Geometry: see drawing. Coordinates: mm, zero at the bounding-box minimum. Round coordinates to 2 decimals unless told otherwise and drop trailing zeros. Loops run counter-clockwise (first coordinate to the right, second up) from the corner with the lowest first, then second, coordinate; pieces in that order, holes last.
(1) Cut plane C-C, the plane z = 28.5. Output: boundary loops of the cut face in (x, y) (1 decimal).
(2) Cut plane D-D, the plane y = 5.25. Output: boundary loops of the cut face in (x, z), and give its area (3 significant figures).
(3) Line query: line 1 (Z direction, x = 2.75, y = 3.75); line 2 (Y direction, x = 3.25, z = 19); line 3 (Y direction, x = 2.5, z = 4) (1 decimal). Output: solid intervals per line, ascending.
(4) First-contact query: pin 1 Ø3 at (x, z) = (2, 12) entering from -Y; pin 2 Ø3 at (x, y) = (3.16, 3.16) entering from +Z; pin 3 Ø1 at (x, y) = (2.5, 3.5) entering from -Z. Flat tips, straight axial feed; report the tip coordinate or a pass-through.
(5) Cut plane B-B, the plane x = 2. Output: boundary loops of the cut face in (y, z), and give its area (3 significant figures).
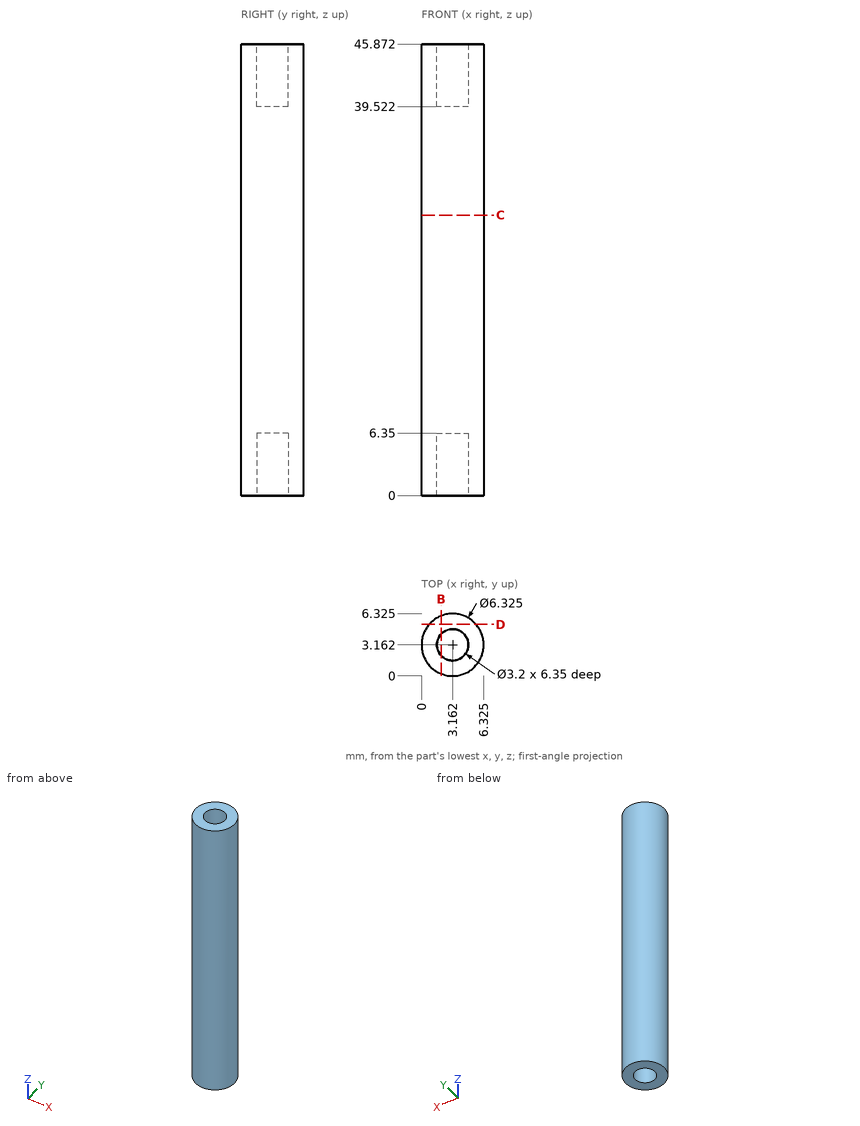
Reported:
1. outline: circle Ø6.3 at (3.2, 3.2)
2. outline: (0.79, 0) - (5.54, 0) - (5.54, 45.87) - (0.79, 45.87) - close
2. area: 218 mm2
3. line 1: z = 6.35 to 39.52
3. line 2: y = 0 to 6.32
3. line 3: y = 0.1 to 1.7, 4.6 to 6.3
4. pin 1: stops at y = 0
4. pin 2: stops at z = 39.52
4. pin 3: stops at z = 6.35
5. outline: (0.22, 0) - (2.06, 0) - (2.06, 6.35) - (4.26, 6.35) - (4.26, 0) - (6.1, 0) - (6.1, 45.87) - (4.26, 45.87) - (4.26, 39.52) - (2.06, 39.52) - (2.06, 45.87) - (0.22, 45.87) - close
5. area: 242 mm2
